Here's how the part is built. I have some questions about the finished solid (model axes, mm). Round coordinates to 2 decimals unless told otherwise and drop trailing zeros. Loops run counter-clockwise (first coordinate to the right, second up) from the corner with the lowest first, then second, coordinate; pieces in that order, holes last. Notation, with made-up numbers: M 72.5,-11 L 128.5,-11 A33 ccw 128.5,27 Z; hole C 56,-37 d11. An arc over 180 degrees is marked long. Write item = value, one per line. Start each with the question number.
Autodesk Inventor part; units mm, degrees
ref_plane "Pracovní rovina16" through (0, 5, 0) normal (0, -1, 0) x (1, 0, 0)
ref_plane "YZ Plane" through (0, 0, 0) normal (1, 0, 0) x (0, 1, 0)
ref_plane "XZ Plane" through (0, 0, 0) normal (0, 1, 0) x (-1, 0, 0)
ref_plane "Pracovní rovina16" through (0, 5, 0) normal (0, -1, 0) x (1, 0, 0)
sketch "Náčrt80" plane through (0, 5, 0) normal (0, -1, 0) x (1, 0, 0)
  circle A0 centre (-22, -24.1875) radius 1.85
  circle A1 centre (22, -24.1875) radius 1.85
  circle A2 centre (-42.25, -8.5) radius 1.85
  circle A3 centre (-42.25, 29) radius 1.85
  circle A4 centre (42.25, -8.5) radius 1.85
  circle A5 centre (42.25, 29) radius 1.85
  arc A6 (-38.75, -8.5) -> (-42.25, -5) centre (-42.25, -8.5) ccw
  line L0 (-45.25, -5) -> (-42.25, -5)
  line L1 (-47.25, -3) -> (-45.25, -5)
  line L2 (-47.25, 23.5) -> (-47.25, -3)
  line L3 (-45.25, 25.5) -> (-47.25, 23.5)
  line L4 (-42.25, 25.5) -> (-45.25, 25.5)
  arc A7 (-42.25, 25.5) -> (-42.25, 32.5) centre (-42.25, 29) ccw
  line L5 (-45.25, 32.5) -> (-42.25, 32.5)
  line L6 (-47.25, 34.5) -> (-45.25, 32.5)
  line L7 (-47.25, 45.3044) -> (-47.25, 34.5)
  line L8 (47.25, 45.3044) -> (-47.25, 45.3044)
  line L9 (47.25, 34.5) -> (47.25, 45.3044)
  line L10 (45.25, 32.5) -> (47.25, 34.5)
  line L11 (42.25, 32.5) -> (45.25, 32.5)
  arc A8 (42.25, 32.5) -> (42.25, 25.5) centre (42.25, 29) ccw
  line L12 (45.25, 25.5) -> (42.25, 25.5)
  line L13 (47.25, 23.5) -> (45.25, 25.5)
  line L14 (47.25, -3) -> (47.25, 23.5)
  line L15 (45.25, -5) -> (47.25, -3)
  line L16 (42.25, -5) -> (45.25, -5)
  arc A9 (42.25, -5) -> (38.75, -8.5) centre (42.25, -8.5) ccw
  arc A10 (31.5, -15.75) -> (38.75, -8.5) centre (31.5, -8.5) ccw
  line L17 (31.5, -15.75) -> (-31.5, -15.75)
  arc A11 (-38.75, -8.5) -> (-31.5, -15.75) centre (-31.5, -8.5) ccw
  line L18 (-5, -41.375) -> (-5, -35.875)
  arc A12 (5, -35.875) -> (-5, -35.875) centre (0, -35.875) ccw
  line L19 (5, -41.375) -> (5, -35.875)
  line L20 (5, -41.375) -> (-5, -41.375)
  arc A13 (-20.6747, -48.0519) -> (-23.3253, -48.0519) centre (-22, -44.8125) ccw
  line L21 (-0.0392, -48.0519) -> (-20.6747, -48.0519)
  line L22 (-2.825, -46.4435) -> (-0.0392, -48.0519)
  line L23 (-2.825, -43.1815) -> (-2.825, -46.4435)
  line L24 (0, -41.5505) -> (-2.825, -43.1815)
  line L25 (2.825, -43.1815) -> (0, -41.5505)
  line L26 (2.825, -46.4435) -> (2.825, -43.1815)
  line L27 (0.0392, -48.0519) -> (2.825, -46.4435)
  line L28 (20.6747, -48.0519) -> (0.0392, -48.0519)
  arc A14 (23.3253, -48.0519) -> (20.6747, -48.0519) centre (22, -44.8125) ccw
  line L29 (27, -48.0519) -> (23.3253, -48.0519)
  line L30 (27, -19.25) -> (27, -48.0519)
  line L31 (49.75, -19.25) -> (27, -19.25)
  line L32 (49.75, 48.4103) -> (49.75, -19.25)
  line L33 (-49.75, 48.4103) -> (49.75, 48.4103)
  line L34 (-49.75, -19.25) -> (-49.75, 48.4103)
  line L35 (-27, -19.25) -> (-49.75, -19.25)
  line L36 (-27, -48.0519) -> (-27, -19.25)
  line L37 (-23.3253, -48.0519) -> (-27, -48.0519)
  line L38 (-31.5, -15.25) -> (31.5, -15.25)
  arc A15 (31.5, -15.25) -> (38.25, -8.5) centre (31.5, -8.5) ccw
  arc A16 (42.25, -4.5) -> (38.25, -8.5) centre (42.25, -8.5) ccw
  line L39 (42.25, -4.5) -> (45.0429, -4.5)
  line L40 (45.0429, -4.5) -> (46.75, -2.7929)
  line L41 (46.75, -2.7929) -> (46.75, 23.2929)
  line L42 (46.75, 23.2929) -> (45.0429, 25)
  line L43 (45.0429, 25) -> (42.25, 25)
  arc A17 (42.25, 33) -> (42.25, 25) centre (42.25, 29) ccw
  line L44 (42.25, 33) -> (45.0429, 33)
  line L45 (45.0429, 33) -> (46.75, 34.7071)
  line L46 (46.75, 34.7071) -> (46.75, 44.8044)
  line L47 (46.75, 44.8044) -> (-46.75, 44.8044)
  line L48 (-46.75, 44.8044) -> (-46.75, 34.7071)
  line L49 (-46.75, 34.7071) -> (-45.0429, 33)
  line L50 (-45.0429, 33) -> (-42.25, 33)
  arc A18 (-42.25, 25) -> (-42.25, 33) centre (-42.25, 29) ccw
  line L51 (-42.25, 25) -> (-45.0429, 25)
  line L52 (-45.0429, 25) -> (-46.75, 23.2929)
  line L53 (-46.75, 23.2929) -> (-46.75, -2.7929)
  line L54 (-46.75, -2.7929) -> (-45.0429, -4.5)
  line L55 (-45.0429, -4.5) -> (-42.25, -4.5)
  arc A19 (-38.25, -8.5) -> (-42.25, -4.5) centre (-42.25, -8.5) ccw
  arc A20 (-38.25, -8.5) -> (-31.5, -15.25) centre (-31.5, -8.5) ccw
  point P0 (0, 0)
  dimension "d487" = 0.5
extrude "Vysunutí84" add sketch "Náčrt80" against normal blind 0.3 contours A20 A19 L55 L54 L53 L52 L51 A18 L50 L49 L48 L47 L46 L45 L44 A17 L43 L42 L41 L40 L39 A16 A15 L38
properties part number "oddělovací plocha"
Item 1: I want a section at B-B, the plane x = -35.5. List the corners of the cut face in (y, z) for me, then the cut area to 3 significant figures.
Item 2: I want a section at A-A, the plane y = 5.1. List the corners of the cut face in (x, z) for me, then the cut area to 3 significant figures.
Item 3: Please list where these lines run through material, in increasing order: line 1 (Z direction, x = -42, y = 5.25); line 2 (Z direction, x = 32, y = 5.25); line 3 (X direction, y = 5.25, z = -6). Write a range as [from, to].
Worked out:
q1.outline = M 5,-13.94 L 5.3,-13.94 L 5.3,44.8 L 5,44.8 Z
q1.area = 17.6 mm2
q2.outline = M -46.75,-2.79 L -45.04,-4.5 L -42.25,-4.5 A4 cw -38.25,-8.5 A6.75 ccw -31.5,-15.25 L 31.5,-15.25 A6.75 ccw 38.25,-8.5 A4 cw 42.25,-4.5 L 45.04,-4.5 L 46.75,-2.79 L 46.75,23.29 L 45.04,25 L 42.25,25 A4 cw 42.25,33 L 45.04,33 L 46.75,34.71 L 46.75,44.8 L -46.75,44.8 L -46.75,34.71 L -45.04,33 L -42.25,33 A4 cw -42.25,25 L -45.04,25 L -46.75,23.29 Z
q2.area = 5,290 mm2
q3.line_1 = [-4.51, 25.01], [32.99, 44.8]
q3.line_2 = [-15.23, 44.8]
q3.line_3 = [-39.13, 39.13]
